CAD build for the part. Positions are in the model's coordinates, mm. A direction names the side the tool comes from. Give positions to 0.01 mm unless a question says otherwise; leave off trailing zeros. Order: outer loops, then holes, each group sorted by start corner. A loop starts at its lowest first (then second) coordinate and runs counter-clockwise, first axis right, second up. Notation, with made-up numbers: (-5, 62.5) -> (40, 62.5) arc R18 ccw to (40, 90.5) -> close; hole circle Ø6 at (15.5, 1.25). An arc over 180 degrees is marked (long way). Use one line per item in the form item = value. Start each with the question number.
1) Probe line 1 (Z direction, x = -11.5, y = -5.25); line 2 (Z direction, x = -9.75, y = -3.75); line 3 (Y direction, x = -1.25, z = -4.75). List the from-to ranges inside material, lowest first.
2) Cut at D-D, the plane z = -1.25. Give the cut face in (x, y), and give its area (3 significant figures).
3) Tool access for faces 1 (the face through (-8.16, 6.257, -3.304)), 2 (the face through (-10.1, 7.7, -0.3)): list every direction of +Z, -Z, +X, -X, +Y, -Y with a clear straight run to the whole face (end or side of a thin tool).
4) Mould opens along Z. For faces 3 (the face through (-0.2, 1.51, -3.13)), 4 (the face through (-3, 0, -6.35)), 5 (the face through (3, 0, 0)), 6 (the face through (-2.24, 10.07, -3.01)) say: pulls with the +Z half, pulls with the -Z half, needs draft (parallel to the pull), parting line crosses it, or undercut.
5) Drop flat-ended pins along their axis: P1, Ø1.8, axis at x = 0, y = 0, coming from the -Z side; P2, Ø2, axis at x = 3, z = -4.5, coming from the -Y side; P3, Ø1.5, axis at x = -3.5, z = -4.5, coming from the +Y side. Give the stop position or say it passes through.
6) Cut at A-A, the plane y = 0. Give the cut face in (x, z) (3 decimals), and give its area (3 significant figures).
7) Cut at C-C, the plane z = -5.25. Give the cut face in (x, y).
from build123d import *

# Parameters (mm, degrees)
SKETCH3_R          = 1.524
CUT_EXTRUDE1_DEPTH = 20.05


with BuildPart() as part:
    # Sketch1 → Revolve1 (revolve)
    with BuildSketch(Plane(origin=(0, 0, 0), x_dir=(0, 0, -1), z_dir=(1, 0, 0)), mode=Mode.PRIVATE) as revolve1_sk:
        Polygon((0, 0), (6.35, 0), (6.35, 12.7), (5.842, 12.7), (3.175, 10.16), (0.508, 12.7), (0, 12.7), align=None)
    revolve(revolve1_sk.sketch.rotate(Axis((0, 0, 0), (0, 0, -1)), 90), axis=Axis((0, 0, 0), (0, 0, -1)))

    # Sketch3 → Cut-Extrude1 (cut, through all)
    with BuildSketch(Plane.XY):
        Circle(SKETCH3_R)
    extrude(amount=-CUT_EXTRUDE1_DEPTH, mode=Mode.SUBTRACT)


solid = part.part
Result:
q1.line_1 = -6.35 to -5.78, -0.57 to 0
q1.line_2 = -6.35 to -3.48, -2.87 to 0
q1.line_3 = -11.59 to -0.87, 0.87 to 11.59
q2.outline = circle Ø23.99 at (0, 0); hole circle Ø3.05 at (0, 0)
q2.area = 445 mm²
q3.face_1 = none
q3.face_2 = +Z, -Z
q4.face_3 = needs draft
q4.face_4 = pulls with the -Z half
q4.face_5 = pulls with the +Z half
q4.face_6 = undercut
q5.P1 = through
q5.P2 = -12.03
q5.P3 = 11.65
q6.outline = (-12.7, -6.35) -> (-1.524, -6.35) -> (-1.524, 0) -> (-12.7, 0) -> (-12.7, -0.508) -> (-10.16, -3.175) -> (-12.7, -5.842) -> close; (1.524, -6.35) -> (12.7, -6.35) -> (12.7, -5.842) -> (10.16, -3.175) -> (12.7, -0.508) -> (12.7, 0) -> (1.524, 0) -> close
q6.area = 128 mm²
q7.outline = circle Ø24.27 at (0, 0); hole circle Ø3.05 at (0, 0)
